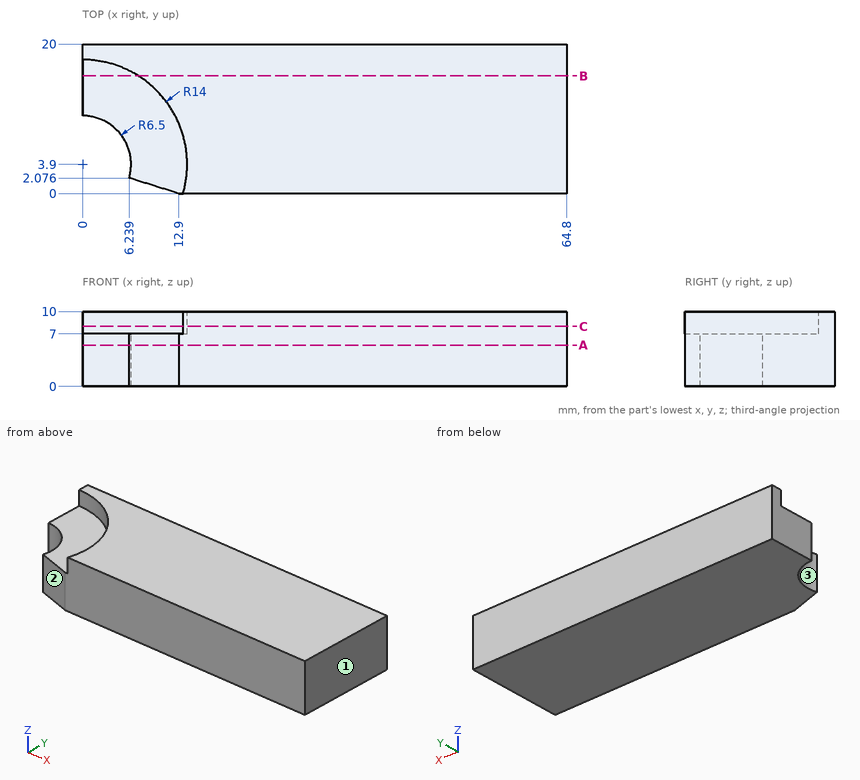
Print and shaded views of the part. All mm, measured from the part's lowest x, y and z. Give positions to 0.01 mm unless a question says otherwise; leave off trailing zeros. Write each loop counter-clockwise with the first axis right and the second up, starting at its lowest first coordinate (ties: lowest second). Pieces come first, ordered by that corner, then holes. Notation, with made-up numbers: (-11, -25) - (10, -25) arc R15 ccw to (10, -19) - close; hole circle Ø4 at (-35.75, 63). An arc over 180 degrees is marked (long way). One line per question, with ' | ' between items. Start each with the question number.
(1) Two-plate mould, pull along Y, no slides. Class the marked faces 1, 2 and 3: +Y half, -Y half, draft (parallel to the pull), parting line (faces both ways), or undercut.
(2) Slice it at B-B on y = 15.75. Write the cut outline in (x, z) (3 decimals), plus the area to 3 significant figures.
(3) Pin check, flat tips, straight feed: P1, Ø11, axis at x = 4, y = 4.5, coming from the +Z side; P2, Ø2, axis at y = 4, z = 1, coming from the -X side. Stop position of each tip, or through.
(4) Slice it at C-C on z = 8. Write the cut outline in (x, y), plus the area to 3 significant figures.
(5) Wall check: line 1 along X through (y, z) = (14, 8.25) (1 decimal); line 2 along Y through (x, z) = (3.5, 4.5); line 3 along Y through (x, z) = (9.5, 8). Give the ranges that are in metal, low to high. Write a range as from..to.
(6) Slice it at A-A on z = 5.5. Write the cut outline in (x, y), plus the area to 3 significant figures.
Results below:
1) face 1: draft | face 2: -Y half | face 3: undercut
2) outline: (0, 0) - (64.8, 0) - (64.8, 10) - (7.455, 10) - (7.455, 7) - (0, 7) - close | area: 626 mm^2
3) P1: z = 7 | P2: x = 6.41
4) outline: (0, 17.9) arc R14 cw to (13.45, 0) - (64.8, 0) - (64.8, 20) - (0, 20) - close | area: 1,090 mm^2
5) line 1: 9.7..64.8 | line 2: 9.38..20 | line 3: 14.18..20
6) outline: (0, 10.4) arc R6.5 cw to (6.24, 2.08) - (12.9, 0) - (64.8, 0) - (64.8, 20) - (0, 20) - close | area: 1,230 mm^2
